Source: three-view drawing plus pictorial views. Frame: mm from the lowest corner of the part. Give positions to 0.01 mm unless a question says otherwise; leave off trailing zeros. Write each loop counter-clockwise with the first axis right and the second up, starting at its lowest first coordinate (ties: lowest second). Pieces come first, ordered by that corner, then holes.
Q1. Cut plane A-A on x = 190. Return the cut outline in (y, z).
Q2. Cut plane C-C on y = 16. Return the cut outline in (x, z), plus the area to 3 significant figures.
Q3. Pin query (flat end, axial travel): pin 1 (1.5 mm diameter, centred on y = 19, z = 0.5, fed in from -X). Return the tip coordinate at first contact, or that it passes through.
Q4. Cut plane B-B on z = 2.5. Return the cut outline in (x, y).
Q5. Line query: L1, parallel to Y at x = 13, z = 1.75; L2, parallel to Y at x = 5, z = 2.15; L3, parallel to Y at x = 100, z = 1.4. Output: solid intervals per line, ascending.
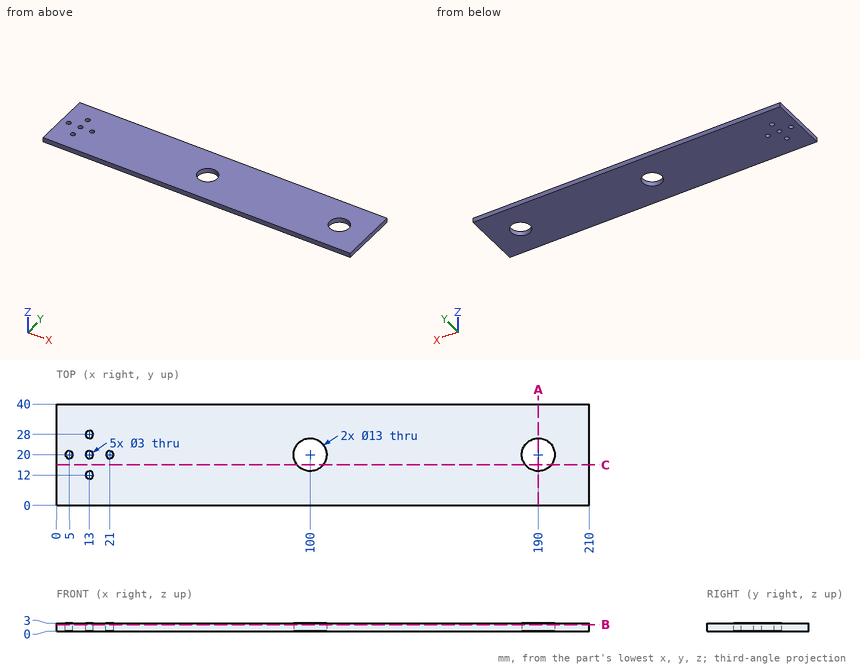
Data:
1. outline: (0, 0) - (13.5, 0) - (13.5, 3) - (0, 3) - close; (26.5, 0) - (40, 0) - (40, 3) - (26.5, 3) - close
2. outline: (0, 0) - (94.88, 0) - (94.88, 3) - (0, 3) - close; (105.12, 0) - (184.88, 0) - (184.88, 3) - (105.12, 3) - close; (195.12, 0) - (210, 0) - (210, 3) - (195.12, 3) - close
2. area: 569 mm2
3. pin 1: stops at x = 0
4. outline: (0, 0) - (210, 0) - (210, 40) - (0, 40) - close; hole circle Ø3 at (5, 20); hole circle Ø3 at (13, 12); hole circle Ø3 at (13, 20); hole circle Ø3 at (13, 28); hole circle Ø3 at (21, 20); hole circle Ø13 at (100, 20); hole circle Ø13 at (190, 20)
5. L1: y = 0 to 10.5, 13.5 to 18.5, 21.5 to 26.5, 29.5 to 40
5. L2: y = 0 to 18.5, 21.5 to 40
5. L3: y = 0 to 13.5, 26.5 to 40
